```python
from build123d import *

# Parameters (mm, degrees)
F1_DEPTH = 7.5
F3_R     = 1
F4_DEPTH = 1.5
F2_R     = 1
F5_DEPTH = 1.5


with BuildPart() as f1:
    # F0 (on Right) → F1 (new body, symmetric)
    with BuildSketch(Plane.YZ):
        with BuildLine():
            Line((-8, 0), (-1.5, 0))
            ThreePointArc((-1.5, 0), (-0.43934, 0.43934), (0, 1.5))
            Line((0, 1.5), (0, 8))
            Line((0, 8), (-1.5, 8))
            Line((-1.5, 8), (-1.5, 2))
            ThreePointArc((-1.5, 2), (-1.646447, 1.646447), (-2, 1.5))
            Line((-2, 1.5), (-8, 1.5))
            Line((-8, 1.5), (-8, 0))
        make_face()
    extrude(amount=F1_DEPTH, both=True)

    # F3 (on face) → F4 (cut)
    with BuildSketch(Plane.XZ.offset(1.5)):
        with Locations((-5, 5)):
            Circle(F3_R)
        with Locations((5, 5)):
            Circle(F3_R)
    extrude(amount=-F4_DEPTH, mode=Mode.SUBTRACT)

    # F2 (on face) → F5 (cut)
    with BuildSketch(Plane.XY.offset(1.5)):
        with Locations((5, -5)):
            Circle(F2_R)
        with Locations((-5, -5)):
            Circle(F2_R)
    extrude(amount=-F5_DEPTH, mode=Mode.SUBTRACT)


solid = f1.part
```
Part model, mm, in its own coordinate system. A direction names the side the tool comes from. Round coordinates to 2 decimals unless told otherwise and drop trailing zeros. Loops run counter-clockwise (first coordinate to the right, second up) from the corner with the lowest first, then second, coordinate; pieces in that order, holes last. Notation, with made-up numbers: (27, 36) -> (43, 36) arc R23 ccw to (43, 68) -> close; hole circle Ø3 at (63, 79). An arc over 180 degrees is marked (long way). Use one line per item in the form item = value. Start each with the question number.
Item 1: Tool access for faces 1 (the flat face through (0, -5, 1.5)), 2 (the cylindrical face through (0.11, -0.45, 0.43)): list every direction of +Z, -Z, +X, -X, +Y, -Y with a clear straight run to the whole face (end or side of a thin tool).
Item 2: Two-plate mould, pull along X, no slides. Class faces 3 (the flat face through (-7.5, -1, 2)), 4 (the cylindrical face through (-5, -1, 6)), 5 (the flat face through (0, -1.5, 5)): released by +X, released by -X, zero draft, split by the parting line, or undercut.
Item 3: Drill centre lines: line 1 along Z through (x, y) = (-0.5, -6.75); line 2 along Z through (x, y) = (5, -0.7); line 3 along Y through (x, z) = (-5, 0.85). Where is each one in solid material? Low to high.
Item 4: Drop flat-ended pins along their axis: pin 1 Ø1 at (x, z) = (1.5, 5.5) entering from -Y; pin 2 Ø2 at (x, y) = (4.5, -7) entering from +Z. Give the stop position or say it passes through.
Item 5: Band-saw the part on C-C (x = -5). List the corners of the cut face in (y, z), plus the area to 3 significant figures.
Item 6: Band-saw the part on D-D (x = -1.5). List the corners of the cut face in (y, z).
Item 7: Band-saw the part on A-A (y = -5). List the corners of the cut face in (x, z), plus the area to 3 significant figures.
Item 8: Band-saw the part on B-B (z = 5). List the corners of the cut face in (x, y).
Data:
q1.face_1 = +Z, +X, -X, -Y
q1.face_2 = -Z, +X, -X, +Y
q2.face_3 = released by -X
q2.face_4 = undercut
q2.face_5 = zero draft
q3.line_1 = 0 to 1.5
q3.line_2 = 0.23 to 4, 6 to 8
q3.line_3 = -8 to -6, -4 to -0.15
q4.pin_1 = -1.5
q4.pin_2 = 1.5
q5.outline = (-8, 0) -> (-6, 0) -> (-6, 1.5) -> (-8, 1.5) -> close; (-4, 0) -> (-1.5, 0) arc R1.5 ccw to (0, 1.5) -> (0, 4) -> (-1.5, 4) -> (-1.5, 2) arc R0.5 cw to (-2, 1.5) -> (-4, 1.5) -> close; (-1.5, 6) -> (0, 6) -> (0, 8) -> (-1.5, 8) -> close
q5.area = 15.3 mm^2
q6.outline = (-8, 0) -> (-1.5, 0) arc R1.5 ccw to (0, 1.5) -> (0, 8) -> (-1.5, 8) -> (-1.5, 2) arc R0.5 cw to (-2, 1.5) -> (-8, 1.5) -> close
q7.outline = (-7.5, 0) -> (-6, 0) -> (-6, 1.5) -> (-7.5, 1.5) -> close; (-4, 0) -> (4, 0) -> (4, 1.5) -> (-4, 1.5) -> close; (6, 0) -> (7.5, 0) -> (7.5, 1.5) -> (6, 1.5) -> close
q7.area = 16.5 mm^2
q8.outline = (-7.5, -1.5) -> (-6, -1.5) -> (-6, 0) -> (-7.5, 0) -> close; (-4, -1.5) -> (4, -1.5) -> (4, 0) -> (-4, 0) -> close; (6, -1.5) -> (7.5, -1.5) -> (7.5, 0) -> (6, 0) -> close
